Input: part model. Units: mm. Frame: model coordinates. A direction names the side the tool comes from. Coordinates: 2 decimals unless noted, no trailing zeros. Order: outer loops, then holes, each group sorted by start corner. A loop starts at its lowest first (then second) coordinate and runs counter-clockwise, first axis right, second up. Notation, with made-up numbers: M -31.5,10 L 11.5,10 A20 ccw 11.5,34 Z; hole C -28,13.5 d1. An arc over 180 degrees is marked long. One line per item, written item: value.
Autodesk Inventor part; units mm, degrees
ref_plane "YZ Plane" through (0, 0, 0) normal (1, 0, 0) x (0, 1, 0)
ref_plane "XZ Plane" through (0, 0, 0) normal (0, 1, 0) x (-1, 0, 0)
ref_plane "XY Plane" through (0, 0, 0) normal (0, 0, 1) x (1, 0, 0)
sketch "草圖1" plane through (0, 0, 0) normal (0, 0, 1) x (1, 0, 0)
  line L0 (25, -10) -> (-25, -10)
  line L1 (-25, -10) -> (-25, 10)
  line L2 (-25, 10) -> (25, 10)
  line L3 (25, 10) -> (25, -10)
  line L4 (25, -10) -> (-25, 10) construction
  line L5 (-25, -10) -> (25, 10) construction
  point P0 (0, 0)
  dimension "d0" = 50
  dimension "d1" = 20
extrude "擠出1" add sketch "草圖1" along normal blind 10
sketch "草圖2" plane through (-25, -10, 0) normal (0, -1, 0) x (1, 0, 0)
  line L0 (0, 10) -> (0, 20)
  line L1 (0, 20) -> (10, 20)
  line L2 (50, 0) -> (50, 10)
  line L3 (0, 10) -> (50, 10)
  line L4 (10, 20) -> (40, 10)
  point P0 (25, 0)
  dimension "d4" = 10
  dimension "d5" = 10
  dimension "d6" = 40
extrude "擠出2" add sketch "草圖2" against normal blind 10
sketch "草圖3" plane through (-25, -10, 0) normal (0, -1, 0) x (1, 0, 0)
  line L0 (0, 0) -> (0, 20)
  line L1 (0, 0) -> (50, 0)
  line L2 (0, 20) -> (10, 20)
  line L3 (10, 20) -> (10, 0)
  line L4 (10, 0) -> (0, 0)
  line L5 (0, 0) -> (0, 20)
  point P0 (25, 0)
  dimension "d9" = 10
extrude "擠出3" add sketch "草圖3" along normal blind 30
fillet "圓角1" radius 10 1 edges at (-20, -40, 20)
sketch "草圖4" plane through (-15, -10, 20) normal (1, 0, 0) x (0, 0, -1)
  circle A0 centre (10, -20) radius 5
  line L0 (20, 0) -> (20, -30)
  line L1 (20, -30) -> (10, -30)
  point P0 (20, 10)
  dimension "d13" = 10
  dimension "d14" = 10
  dimension "d15" = 10
extrude "擠出4" cut sketch "草圖4" against normal blind 30
sketch "草圖5" plane through (-25, 0, 0) normal (0, 1, 0) x (1, 0, 0)
  line L0 (0, -20) -> (0, -10)
  line L1 (0, -10) -> (0, -50)
  line L2 (49.7047, -10) -> (49.7047, -40)
  line L3 (49.7047, -40) -> (20, -50)
  line L4 (20, -50) -> (0, -50)
  line L5 (50, -10) -> (0, -10)
  circle A0 centre (39.7047, -30) radius 5
  point P0 (25, 0)
  dimension "d18" = 40
  dimension "d19" = 30
  dimension "d20" = 20
  dimension "d21" = 10
  dimension "d22" = 20
  dimension "d23" = 10
extrude "擠出5" add sketch "草圖5" along normal blind 10
properties part number "件30"
(1) Cut plane D-D on y = -28.5. Output: boundary loops of the cut face in (x, z), plus the area to 3 significant figures.
Data:
outline: M -25,0 L -15,0 L -15,5.23 L -25,5.23 Z; M -25,14.77 L -15,14.77 L -15,20 L -25,20 Z
area: 105 mm2
(2) Cut plane C-C on y = 6.5. Output: boundary loops of the cut face in (x, z), plus the area to 3 significant figures.
Data:
outline: M -25,0 L 25,0 L 25,10 L 24.7,10 L 24.7,40 L -5,50 L -25,50 Z; hole C 14.7,30 d10
area: 2,260 mm2
(3) First-contact query: pin 1 (6 mm diameter, centred on x = -11, z = 28.5, fed in from -Y); pin 2 (8 mm diameter, centred on x = 21, y = -3.5, fed in from +Z); pin 3 (22 mm diameter, centred on y = -18.5, z = 10.5, fed in from +X); pin 4 (8 mm diameter, centred on x = -20, y = -15, fed in from +Z). Flat tips, straight axial feed; report the tip coordinate or a pass-through.
Data:
pin 1: stops at y = 0
pin 2: stops at z = 41.9
pin 3: stops at x = 25
pin 4: stops at z = 20
(4) Cut plane B-B on x = -16.5. Output: boundary loops of the cut face in (y, z), plus the area to 3 significant figures.
Data:
outline: M -40,0 L 10,0 L 10,50 L 0,50 L 0,20 L -30,20 A10 ccw -40,10 Z; hole C -30,10 d10
area: 1,200 mm2
(5) Cut plane A-A on z = 30. Output: boundary loops of the cut face in (x, y).
Data:
outline: M -25,0 L 9.7,0 L 9.7,10 L -25,10 Z; M 19.7,0 L 24.7,0 L 24.7,10 L 19.7,10 Z
(6) Ray query, line 1 (X direction, y = 2, z = 30); line 2 (Y direction, x = -22.5, z = 10); line 3 (Y direction, x = 2, z = 37). Return the intervals inside material, ascending. Write a range as from..to.
Data:
line 1: x = -25..9.7, 19.7..24.7
line 2: y = -40..-35, -25..10
line 3: y = 0..10
(7) Access query for faces 1 (the cylindrical face through (-19.93, -36.99, 17.15)), 2 (the flat face through (0, -5, 15)), 3 (the flat face through (1, -10, 8)), 4 (the flat face through (-25, -9.8, 19.8)), 5 (the flat face through (24.705, 5, 25)). Directions: +Z, -Z, +X, -X, +Y, -Y. A direction counts if a zero-diameter tool reaches every point of the face in a straight line with its end or side. Return the directions, or none.
Data:
face 1: +Z, +X, -X, -Y
face 2: +Z, +X, -Y
face 3: +Z, -Z, +X, -Y
face 4: +Z, -Z, -X, +Y, -Y
face 5: +Z, +X, +Y, -Y
(8) Draft query along Z for faces 6 (the flat face through (0, 0, 30)), 7 (the flat face through (-20, -15, 20)), 8 (the cylindrical face through (-19.93, -31.915, 5.381)). Return one class per face: released by +Z, released by -Z, zero draft, split by the parting line, or undercut.
Data:
face 6: zero draft
face 7: released by +Z
face 8: undercut
